Here's how the part is built. I have some questions about the finished solid (model axes, mm). A direction names the side the tool comes from. Coordinates: 2 decimals unless noted, no trailing zeros. Write each loop counter-clockwise with the first axis right and the second up, starting at its lowest first coordinate (ties: lowest second). Pieces come first, ordered by that corner, then holes.
from build123d import *

# Parameters (mm, degrees)
SCHIZZO1_R                   = 15
ESTRUSIONE_ESTRUSIONE1_DEPTH = 30
SCHIZZO3_R                   = 5.75
TAGLIO_ESTRUSIONE1_DEPTH     = 2
SCHIZZO4_R                   = 13.25
TAGLIO_ESTRUSIONE2_DEPTH     = 36.128336141
ESTRUSIONE_ESTRUSIONE2_START = -5
ESTRUSIONE_ESTRUSIONE2_DEPTH = 5
RACCORDO1_R                  = 5


with BuildPart() as part:
    # Schizzo1 → Estrusione-Estrusione1 (new body)
    with BuildSketch(Plane(origin=(0, 0, 0), x_dir=(1, 0, 0), z_dir=(0, 1, 0))):
        with Locations(Location((0, 0, 0), (0, 0, 270))):
            Circle(SCHIZZO1_R)
    extrude(amount=ESTRUSIONE_ESTRUSIONE1_DEPTH)

    # Schizzo3 → Taglio-Estrusione1 (cut)
    with BuildSketch(Plane.XZ):
        with Locations(Location((0, 0, 0), (0, 0, 270))):
            Circle(SCHIZZO3_R)
    extrude(amount=-TAGLIO_ESTRUSIONE1_DEPTH, mode=Mode.SUBTRACT)

    # Schizzo4 → Taglio-Estrusione2 (cut, through all)
    with BuildSketch(Plane.XZ.offset(-2)):
        with Locations(Location((0, 0, 0), (0, 0, 270))):
            Circle(SCHIZZO4_R)
    extrude(amount=-TAGLIO_ESTRUSIONE2_DEPTH, mode=Mode.SUBTRACT)

    # Schizzo5 → Estrusione-Estrusione2 (add)
    with BuildSketch(Plane(origin=(0, 30, 0), x_dir=(1, 0, 0), z_dir=(0, 1, 0)).offset(ESTRUSIONE_ESTRUSIONE2_START)):
        with BuildLine():
            Line((-13.164820546, 1.5), (-9.127568132, 1.5))
            ThreePointArc((-9.127568132, 1.5), (-9.25, 0), (-9.127568132, -1.5))
            Line((-9.127568132, -1.5), (-13.164820546, -1.5))
            ThreePointArc((-13.164820546, -1.5), (-13.25, 0), (-13.164820546, 1.5))
        make_face()
    extrude(amount=ESTRUSIONE_ESTRUSIONE2_DEPTH)

    # Raccordo1
    raccordo1_edges = [part.edges().sort_by_distance(p)[0] for p in [
        (0, 0, -15),
    ]]
    fillet(raccordo1_edges, radius=RACCORDO1_R)


solid = part.part
1. I want a section at C-C (y = 7.25). List the corners of the cut face in (x, z) for me, then the cut area to 3 significant figures.
2. I want a section at A-A (z = 0). List the corners of the cut face in (x, y) for me.
3. For pin 1 Ø1.5 at (x, y) = (3, 4.5) entering from +Z; pin 2 Ø8 at (y, z) = (8.5, 12) entering from +X; pin 3 Ø3 at (x, y) = (10.5, 18) entering from +Z; pin 4 Ø10.5 at (x, z) = (0, 0) entering from +Y, each with a flat end and sliding along its axis, tell me the tip position at first contact or that it passes through.
4. If I drill on line 1 (X direction, y = 12.75, z = 0.5); line 2 (Z direction, x = -9.75, y = 9.5); line 3 (Z direction, x = 8, y = 27.5), over which ranges is the centre line in solid material (lowest first)?
5. I want a section at B-B (x = 0). List the corners of the cut face in (y, z) for me, then the cut area to 3 significant figures.
6. I want a section at D-D (y = 3.25). List the corners of the cut face in (x, z) for me.
7. On a 3-axis mill with a long thin cutter (end or side, diameter ignored), from which of +Z, -Z, +X, -X, +Y, -Y can I reach the whole of each face in a straight line? I mean faces 1 (the face through (-11, 25, 0)), 2 (the face through (-4.3, 0, 4.3)), 3 (the face through (-9.25, 27.46, -0.02)). Say none if no direction works.
8. Thinking about a two-plate mould opening in Z: for faces 4 (the face through (4.85, 0.99, -3.09)), 5 (the face through (-10, 30, 0)), 6 (the face through (0.66, 17.325, -14.985)), which applies, pulls with the +Z half, pulls with the -Z half, needs draft (parallel to the pull), parting line crosses it, or undercut?
Response values:
1. outline: circle Ø30 at (0, 0); hole circle Ø26.5 at (0, 0)
1. area: 155 mm2
2. outline: (-15, 5) arc R5 ccw to (-10, 0) - (-5.75, 0) - (-5.75, 2) - (-13.25, 2) - (-13.25, 25) - (-9.25, 25) - (-9.25, 30) - (-15, 30) - close; (5.75, 0) - (10, 0) arc R5 ccw to (15, 5) - (15, 30) - (13.25, 30) - (13.25, 2) - (5.75, 2) - close
3. pin 1: stops at z = 14.82
3. pin 2: stops at x = 12.69
3. pin 3: stops at z = 12
3. pin 4: passes through
4. line 1: x = -14.99 to -13.24, 13.24 to 14.99
4. line 2: z = -11.4 to -8.97, 8.97 to 11.4
4. line 3: z = -12.69 to -10.56, 10.56 to 12.69
5. outline: (0, -10) arc R5 ccw to (5, -15) - (30, -15) - (30, -13.25) - (2, -13.25) - (2, -5.75) - (0, -5.75) - close; (0, 5.75) - (2, 5.75) - (2, 13.25) - (30, 13.25) - (30, 15) - (5, 15) arc R5 ccw to (0, 10) - close
5. area: 124 mm2
6. outline: circle Ø29.37 at (0, 0); hole circle Ø26.5 at (0, 0)
7. face 1: none
7. face 2: +Z, -Z, +X, -X, -Y
7. face 3: +Y
8. face 4: undercut
8. face 5: needs draft
8. face 6: parting line crosses it
